Part model, mm, in its own coordinate system. Face numbers are marked on the shaded views. Round coordinates to 2 decimals unless told otherwise and drop trailing zeros. Loops run counter-clockwise (first coordinate to the right, second up) from the corner with the lowest first, then second, coordinate; pieces in that order, holes last.
Autodesk Inventor part; units mm, degrees
ref_plane "YZ Plane" through (0, 0, 0) normal (1, 0, 0) x (0, 1, 0)
ref_plane "XZ Plane" through (0, 0, 0) normal (0, 1, 0) x (-1, 0, 0)
ref_plane "XY Plane" through (0, 0, 0) normal (0, 0, 1) x (1, 0, 0)
sketch "Sketch1" plane through (0, 0, 0) normal (0, 0, 1) x (1, 0, 0)
  point P0 (0, 0)
sketch "Sketch2" plane through (0, 0, 0) normal (0, 1, 0) x (-1, 0, 0)
  point P0 (0, 0)
sketch "Sketch3" plane through (0, 0, 0) normal (0, 0, 1) x (1, 0, 0)
  point P0 (0, 0)
sketch "Sketch4" plane through (0, 0, 0) normal (0, 1, 0) x (-1, 0, 0)
  line L0 (33, 1) -> (0, 1)
  line L1 (0, 1) -> (0, -24)
  line L2 (0, -24) -> (33, -24)
  line L3 (33, -24) -> (33, 1)
  dimension "d0" = 33
  dimension "d2" = 25
extrude "Extrusion1" add sketch "Sketch4" along normal blind 2
sketch "Sketch8" plane through (0, 2, 0) normal (0, 1, 0) x (1, 0, 0)
  line L0 (-0.0049, 24) -> (-32.9741, 24)
  line L1 (0, 0) -> (-2, 0)
  line L2 (-2, 0) -> (-2, 24)
  line L3 (-2, 24) -> (0, 24)
  line L4 (0, 24) -> (0, 0)
  dimension "d18" = 2
sketch "Sketch13" plane through (0, 2, 0) normal (0, 1, 0) x (1, 0, 0)
  point P0 (0, 0)
sketch "Sketch14" plane through (0, 2, 0) normal (0, 1, 0) x (1, 0, 0)
  point P0 (0, 0)
extrude "Extrusion9" add sketch "Sketch8" along normal blind 8
sketch "Sketch15" plane through (0, 2, 0) normal (0, 1, 0) x (1, 0, 0)
  line L0 (-33, -1) -> (0, -1)
  line L1 (0, -1) -> (0, 1)
  line L2 (0, 1) -> (-33, 1)
  line L3 (-33, 1) -> (-33, -1)
  point P0 (0, 0)
  dimension "d32" = 2
extrude "Extrusion10" add sketch "Sketch15" along normal blind 8
sketch "Sketch16" plane through (0, 2, 0) normal (0, 1, 0) x (1, 0, 0)
  line L0 (0, 0) -> (0, 24)
  line L1 (-33, 24) -> (0, 24)
  line L2 (0, 24) -> (0, 21.9991)
  line L3 (0, 21.9991) -> (-33, 21.9991)
  line L4 (-33, 21.9991) -> (-33, 24)
extrude "Extrusion11" add sketch "Sketch16" along normal blind 8
sketch "Sketch17" plane through (0, 2, 0) normal (0, 1, 0) x (1, 0, 0)
  line L0 (0, 24) -> (-33, 24)
  line L1 (-33, -1) -> (-31.0023, -1)
  line L2 (-31.0023, -1) -> (-31.0023, 24)
  line L3 (-31.0023, 24) -> (-33, 24)
  line L4 (-33, 24) -> (-33, -1)
  point P0 (0, 0)
extrude "Extrusion12" add sketch "Sketch17" along normal blind 8
sketch "Sketch18" plane through (-31.0023, 2, -1) normal (1, 0, 0) x (0, 0, -1)
  line L0 (23, -2) -> (23, 8)
  line L1 (-2, 8) -> (23, 8)
  line L2 (23, 8) -> (23, 5.9835)
  line L3 (23, 5.9835) -> (-2, 5.9835)
  line L4 (-2, 5.9835) -> (-2, 8)
  point P0 (-1, -2)
extrude "Extrusion13" add sketch "Sketch18" along normal blind 2
sketch "Sketch19" plane through (0, 0, 1) normal (1, 0, 0) x (0, 0, -1)
  point P0 (1, 0)
sketch "Sketch20" plane through (0, 0, 1) normal (1, 0, 0) x (0, 0, -1)
  circle A0 centre (5, 6) radius 1.5
  line L0 (0, 0) -> (25, 0)
  line L1 (0, 0) -> (0, 10)
  circle A1 centre (8, 6) radius 1.5
  circle A2 centre (11, 6) radius 1.4979
  circle A3 centre (14, 6) radius 1.5
  circle A4 centre (17, 6) radius 1.5
  circle A5 centre (20, 6) radius 1.5
  line L2 (25, 0) -> (25, 10)
  point P0 (1, 0)
  dimension "d41" = 6
  dimension "d42" = 5
  dimension "d43" = 3
  dimension "d44" = 3
  dimension "d45" = 3
  dimension "d46" = 3
  dimension "d47" = 3
  dimension "d48" = 3
  dimension "d49" = 3
  dimension "d50" = 3
  dimension "d51" = 3
  dimension "d52" = 3
  dimension "d60" = 5
hole "Hole1" at (0, 6, -4) at (0, 6, -7) at (0, 6, -10) at (0, 6, -13) at (0, 6, -16) at (0, 6, -19) direction (-1, 0, 0) diameter 3 depth 2 tip angle 118
sketch "Sketch21" plane through (-2, 2, -1) normal (-1, 0, 0) x (0, 0, 1)
  point P0 (1, -2)
sketch "Sketch22" plane through (-2, 2, -1) normal (-1, 0, 0) x (0, 0, 1)
  point P0 (1, -2)
sketch "Sketch23" plane through (0, 0, 1) normal (1, 0, 0) x (0, 0, -1)
  line L0 (5, 7) -> (20.6591, 7)
  line L1 (20.6591, 7) -> (20.6591, 5)
  line L2 (20.6591, 5) -> (5, 5)
  line L3 (5, 5) -> (5, 7)
  arc A0 (12.5, 6) -> (9.5, 6) centre (11, 6) ccw
  arc A1 (9.5, 6) -> (12.5, 6) centre (11, 6) ccw
  point P0 (1, 0)
  dimension "d62" = 0.5
  dimension "d64" = 0.5
extrude "Extrusion14" cut sketch "Sketch23" against normal blind 9.525 contours L0 A0 A1 L2 L3 | L0 A0 A1 L2 | L0 L1 L2 A1 A0
sketch "Sketch24" plane through (0, 0, 0) normal (0, -1, 0) x (1, 0, 0)
  point P0 (0, 0)
sketch "Sketch26" plane through (0, 0, 0) normal (0, -1, 0) x (1, 0, 0)
  point P0 (0, 0)
sketch "Sketch27" plane through (0, 0, 0) normal (0, -1, 0) x (1, 0, 0)
  circle A0 centre (-17.6464, -11.4968) radius 10
  line L0 (-33, 1) -> (0, 1)
  line L1 (0, -24) -> (-33, -24)
  point P0 (0, 0)
  dimension "d69" = 20
  dimension "d70" = 12.4968
  dimension "d71" = 12.5032
hole "Hole2" at (-17.6464, 0, -11.4968) direction (0, 1, 0) diameter 20 depth 2 tip angle 118
properties part number "Sensor_Bracket"
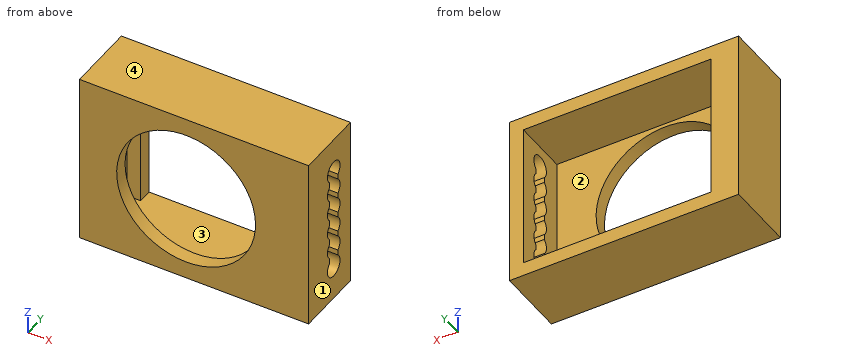
1) Slice it at A-A, the plane z = -3.75. Give the cut face in (x, y), then the cut area to 3 significant figures.
Values:
outline: (-33, 0) - (-23.97, 0) - (-23.97, 2) - (-31, 2) - (-31, 7.98) - (-29, 7.98) - (-29, 10) - (-33, 10) - close; (-11.32, 0) - (0, 0) - (0, 4.52) - (-2, 4.52) - (-2, 2) - (-11.32, 2) - close; (-2, 7.48) - (0, 7.48) - (0, 10) - (-2, 10) - close
area: 70.8 mm2
2) Mould opens along X. For the marked faces 1, 2, 3 and 4 say: released by +X, released by -X, zero draft, split by the parting line, or undercut.
Values:
face 1: released by +X
face 2: undercut
face 3: undercut
face 4: zero draft
3) Drop flat-ended pins along their axis: pin 1 Ø1 at (x, z) = (-30, -10) entering from -Y; pin 2 Ø8 at (x, z) = (-9, -14.5) entering from +Y. Give the stop position or say it passes through.
Values:
pin 1: stops at y = 0
pin 2: stops at y = 2
4) Slice it at B-B, the plane y = 8.75. Give the cut face in (x, z).
Values:
outline: (-33, -24) - (0, -24) - (0, 1) - (-33, 1) - close; hole (-29, -22) - (-2, -22) - (-2, -1) - (-29, -1) - close
5) Slice it at C-C, the plane x = -15. Give the cut face in (y, z), then the cut area to 3 significant figures.
Values:
outline: (0, -24) - (10, -24) - (10, -22) - (2, -22) - (2, -21.14) - (0, -21.14) - close; (0, -1.85) - (2, -1.85) - (2, -1) - (10, -1) - (10, 1) - (0, 1) - close
area: 43.4 mm2
6) Wall check: line 1 along Z through (x, y) = (-0.55, 6); line 2 along Z through (x, y) = (-26, 5); line 3 along Y through (x, z) = (-30, -7.75). Give the ranges that are in metal, low to high.
Values:
line 1: z = -24 to -20.5, -2.5 to 1
line 2: z = -24 to -22, -1 to 1
line 3: y = 0 to 2, 7.98 to 10
7) Slice it at D-D, the plane y = 6. Give the cut face in (x, z), then the cut area to 3 significant figures.
Values:
outline: (-33, -24) - (0, -24) - (0, -20.5) - (-2, -20.5) - (-2, -22) - (-31, -22) - (-31, -1) - (-2, -1) - (-2, -2.5) - (0, -2.5) - (0, 1) - (-33, 1) - close
area: 180 mm2
